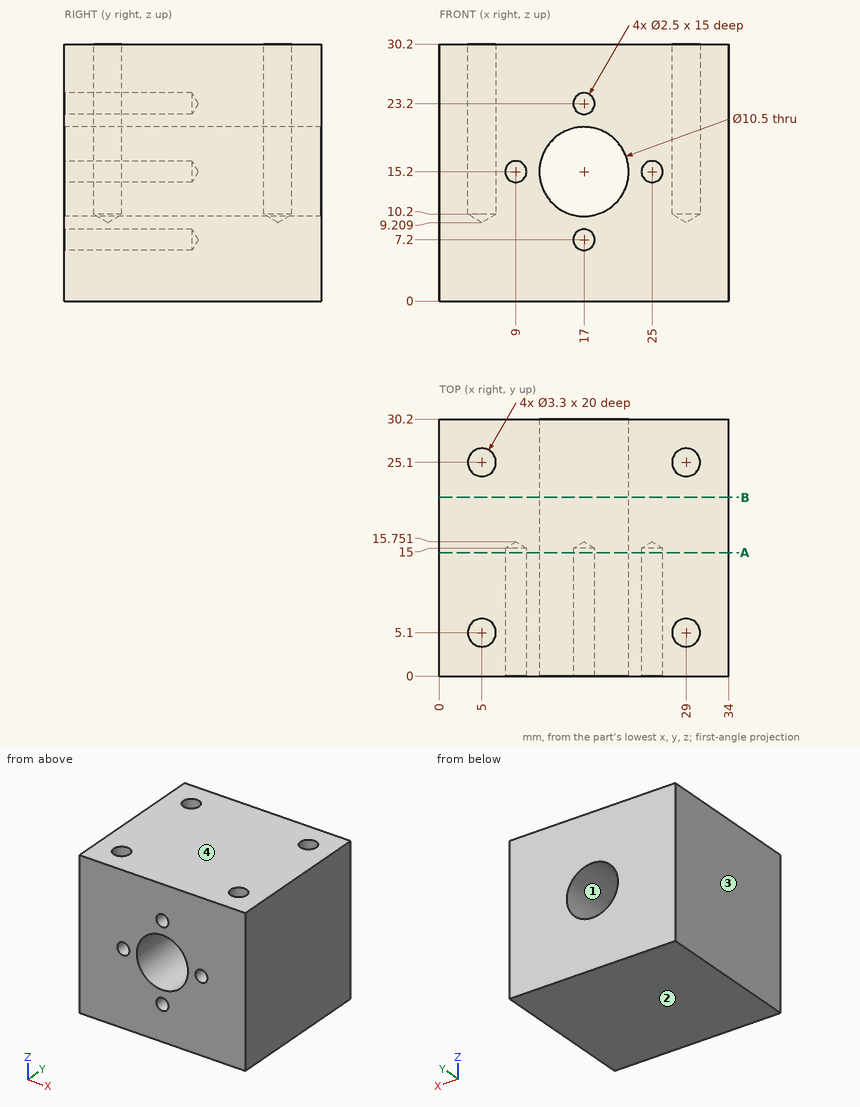
Check sheet for the drawn part. Datum: minimum x, y, z corner. Units: mm. Round coordinates to 2 decimals unless told otherwise and drop trailing zeros. Write each loop counter-clockwise with the first axis right and the second up, starting at its lowest first coordinate (ties: lowest second). Pieces come first, ordered by that corner, then holes. Notation, with made-up numbers: (32, -37.75) - (90, -37.75) arc R33 cw to (90, -0.75) - close; hole circle Ø8 at (55, 43.25). An arc over 180 degrees is marked (long way). Return JSON: item names as keys, results as strings.
Q1. Depth check by flat-ended pin: P1, Ø2, axis at x = 5, y = 25.1, coming from the +Z side; P2, Ø9.5, axis at x = 17, z = 15.2, coming from the -Y side; P3, Ø1.5, axis at x = 17, z = 23.2, coming from the -Y side. Enter the tip coordinate at first touch or a pass-through.
Returned:
{"P1": "stops at z = 9.81", "P2": "passes through", "P3": "stops at y = 15.3"}
Q2. Cross-section at A-A (y = 14.5). Record the boundary of the cut face in (x, z).
Returned:
{"outline": "(0, 0) - (34, 0) - (34, 30.2) - (0, 30.2) - close; hole circle Ø2.5 at (9, 15.2); hole circle Ø10.5 at (17, 15.2); hole circle Ø2.5 at (17, 7.2); hole circle Ø2.5 at (17, 23.2); hole circle Ø2.5 at (25, 15.2)"}
Q3. Cross-section at B-B (y = 21). Record the boundary of the cut face in (x, z), then the cut area to 3 significant figures.
Returned:
{"outline": "(0, 0) - (34, 0) - (34, 30.2) - (0, 30.2) - close; hole circle Ø10.5 at (17, 15.2)", "area": "940 mm²"}
Q4. Scan lines: L1, parallel to X at y = 25, z = 15; L2, parallel to Z at x = 17, y = 13.5; L3, parallel to Y at x = 5, z = 21.75. Record each from-to range of solid material in increasing order. Write a range as from..to.
Returned:
{"L1": "x = 0..3.35, 6.65..11.75, 22.25..27.35, 30.65..34", "L2": "z = 0..5.95, 8.45..9.95, 20.45..21.95, 24.45..30.2", "L3": "y = 0..3.45, 6.75..23.45, 26.75..30.2"}
Q5. Draft check along Z on the marked faces 1, 2, 3 and 4. Enter one of: released by +Z, released by -Z, zero draft, split by the parting line, or undercut.
Returned:
{"face 1": "undercut", "face 2": "released by -Z", "face 3": "zero draft", "face 4": "released by +Z"}
